The listing builds one solid part. Answer for the finished solid, in the listing's coordinates (mm). A direction names the side the tool comes from. Give positions to 0.01 mm unless a question says otherwise; leave off trailing zeros. Loops run counter-clockwise (first coordinate to the right, second up) from the corner with the lowest first, then second, coordinate; pieces in that order, holes last. Notation, with made-up numbers: (44, 66.25) - (87, 66.25) arc R22 ccw to (87, 101.25) - close; hole circle Ø2 at (-35.75, 68.25). An arc over 180 degrees is marked (long way). Answer in a Markdown table with one row per item. Add a question column.
```python
from build123d import *

# Parameters (mm, degrees)
F1_DEPTH = 25


with BuildPart() as f1:
    # F0 (on Front) → F1 (new body)
    with BuildSketch(Plane.XZ):
        with BuildLine():
            Line((28.859725, 5.826163), (13.71945, 23.652325))
            ThreePointArc((13.71945, 23.652325), (7.558378, 28.336185), (0, 30))
            ThreePointArc((0, 30), (-7.558378, 28.336185), (-13.71945, 23.652325))
            Line((-13.71945, 23.652325), (-28.859725, 5.826163))
            ThreePointArc((-28.859725, 5.826163), (-30.911458, -1.259331), (-26.976691, -7.498836))
            Line((-26.976691, -7.498836), (-6.635588, -20.998449))
            ThreePointArc((-6.635588, -20.998449), (-3.465445, -22.48872), (0, -23))
            ThreePointArc((0, -23), (3.465445, -22.48872), (6.635588, -20.998449))
            Line((6.635588, -20.998449), (26.976691, -7.498836))
            ThreePointArc((26.976691, -7.498836), (30.911458, -1.259331), (28.859725, 5.826163))
        make_face()
        with BuildLine():
            Line((15, 12.87607), (15, 5.656854))
            ThreePointArc((15, 5.656854), (13, 0), (15, -5.656854))
            Line((15, -5.656854), (15, -8.246191))
            Line((15, -8.246191), (3.317794, -15.999224))
            ThreePointArc((3.317794, -15.999224), (1.732722, -16.74436), (0, -17))
            ThreePointArc((0, -17), (-1.732722, -16.74436), (-3.317794, -15.999224))
            Line((-3.317794, -15.999224), (-15, -8.246191))
            Line((-15, -8.246191), (-15, -5.656854))
            ThreePointArc((-15, -5.656854), (-13, 0), (-15, 5.656854))
            Line((-15, 5.656854), (-15, 12.87607))
            Line((-15, 12.87607), (-9.1463, 19.768217))
            ThreePointArc((-9.1463, 19.768217), (-5.038918, 22.89079), (0, 24))
            ThreePointArc((0, 24), (5.038918, 22.89079), (9.1463, 19.768217))
            Line((9.1463, 19.768217), (15, 12.87607))
        make_face(mode=Mode.SUBTRACT)
    extrude(amount=F1_DEPTH)


solid = f1.part
```
(1) A tool of negligible diameter and unlimited length cuts with its end or side. For faces 4 (the face through (-30.926, -12.325, -1.154)), 5 (the face through (9.24, -12.32, -12.07)), from which of +Z, -Z, +X, -X, +Y, -Y can it reach the whole face along a straight path? Write none if from no direction.
(2) Given pin 1 Ø1 at (y, z) = (-5.5, -17) entering from -X; pin 2 Ø5 at (y, z) = (-6.5, 15.5) entering from +X; pin 3 Ø2 at (y, z) = (-15, -8) entering from +X; pin 4 Ø4 at (x, z) = (24.5, -13) entering from -Y, each flat-ended and moving along its own axis, determine where each tip first touches the part or whether it passes through.
(3) A cutting plane is placed at A-A on y = -21. Determine the outline of the cut face in (x, z).
(4) A cutting plane is placed at D-D on x = -19. Determine the outline of the cut face in (y, z) (3 decimals).
(5) The mould has two halves that part along Z. Classify faces 1 (the face through (12.03, -12.32, 16.37)), 2 (the face through (-14.2, 0, 3.9)), 3 (the face through (30.896, -12.325, -1.365)): pulls with the +Z half, pulls with the -Z half, needs draft (parallel to the pull), parting line crosses it, or undercut.
(6) A cutting plane is placed at B-B on z = -4.5. Determine the outline of the cut face in (x, y).
(7) A cutting plane is placed at C-C on x = -1.5. Determine the outline of the cut face in (y, z).
(8) Find the intervals of material crossed by line 1 along X through (y, z) = (-2.5, 2.5); line 2 along X through (y, z) = (-5.25, -13.5); line 3 along Z through (x, y) = (-5, -15), in increasing order. Write a range as [from, to].
Evaluation:
| question | item | result |
|---|---|---|
| 1 | face 4 | -X, +Y, -Y |
| 1 | face 5 | +Y, -Y |
| 2 | pin 1 | stops at x = -13.41 |
| 2 | pin 2 | stops at x = 22.77 |
| 2 | pin 3 | stops at x = 27.66 |
| 2 | pin 4 | passes through |
| 3 | outline | (-28.86, 5.83) arc R9 ccw to (-26.98, -7.5) - (-6.64, -21) arc R12 ccw to (0, -23) arc R12 ccw to (6.64, -21) - (26.98, -7.5) arc R9 ccw to (28.86, 5.83) - (13.72, 23.65) arc R18 ccw to (0, 30) arc R18 ccw to (-13.72, 23.65) - close; hole (-15, -8.25) - (-3.32, -16) arc R6 ccw to (0, -17) arc R6 ccw to (3.32, -16) - (15, -8.25) - (15, -5.66) arc R9 cw to (15, 5.66) - (15, 12.88) - (9.15, 19.77) arc R12 ccw to (-9.15, 19.77) - (-15, 12.88) - (-15, 5.66) arc R9 cw to (-15, -5.66) - close |
| 4 | outline | (-25, -12.793) - (0, -12.793) - (0, 17.435) - (-25, 17.435) - close |
| 5 | face 1 | undercut |
| 5 | face 2 | needs draft |
| 5 | face 3 | parting line crosses it |
| 6 | outline | (-29.79, -25) - (-14.21, -25) - (-14.21, 0) - (-29.79, 0) - close; (14.21, -25) - (29.79, -25) - (29.79, 0) - (14.21, 0) - close |
| 7 | outline | (-25, -22.91) - (0, -22.91) - (0, -16.81) - (-25, -16.81) - close; (-25, 23.91) - (0, 23.91) - (0, 29.94) - (-25, 29.94) - close |
| 8 | line 1 | x = [-30.65, -13.35], [13.35, 30.65] |
| 8 | line 2 | x = [-17.93, -7.08], [7.08, 17.93] |
| 8 | line 3 | z = [-21.91, -14.88], [22.91, 29.29] |
